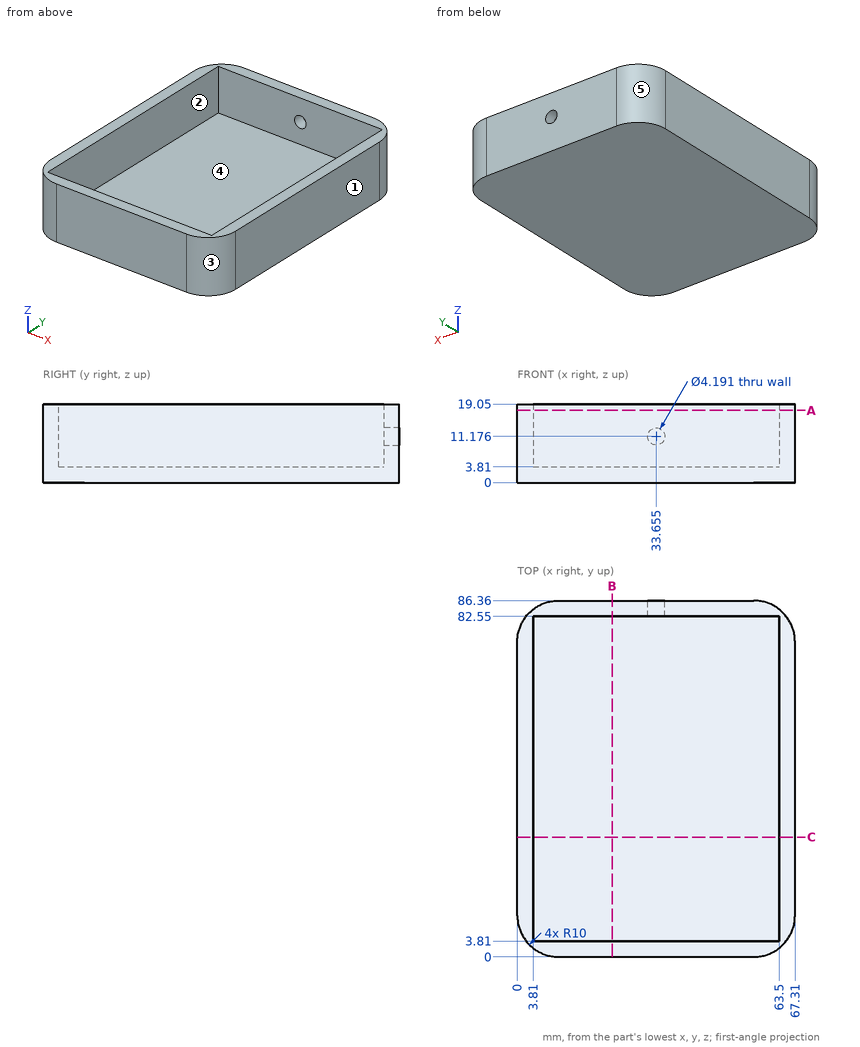
Can you work these out from the drawing? Everything is in mm from the part's minimum corner. A direction names the side the tool comes from. Round coordinates to 2 decimals unless told otherwise and drop trailing zeros. Write each loop counter-clockwise with the first axis right and the second up, starting at its lowest first coordinate (ties: lowest second). Pieces come first, ordered by that corner, then holes.
1. For the marked faces 1 and 2, which set-ups out of +Z, -Z, +X, -X, +Y, -Y let a thin tool reach every point of the face, with its end or its side?
2. Suppose I cut it at B-B (x = 23). List the corners of the cut face in (y, z) for me, and give its area (3 significant figures).
3. Suppose I cut it at A-A (z = 17.5). List the corners of the cut face in (x, y) for me, and give its area (3 significant figures).
4. If we mould it in two halves opening along X, with no side actions, what happens to the marked faces 3, 4 and 5? For each: released by +X, released by -X, zero draft, split by the parting line, or undercut.
5. I need wall thicknesses on L1, parallel to Y at x = 54, z = 18.25; L2, parallel to X at y = 74.5, z = 8; L3, parallel to Z at x = 58, y = 33. Which ranges of each line are inside material? Lowest first, please.
6. Suppose I cut it at C-C (y = 29). List the corners of the cut face in (x, z) for me, and give its area (3 significant figures).
Answer sheet:
1. face 1: +Z, -Z, +X, +Y, -Y
1. face 2: +Z
2. outline: (0, 0) - (86.36, 0) - (86.36, 19.05) - (82.55, 19.05) - (82.55, 3.81) - (3.81, 3.81) - (3.81, 19.05) - (0, 19.05) - close
2. area: 445 mm2
3. outline: (0, 10) arc R10 ccw to (10, 0) - (57.31, 0) arc R10 ccw to (67.31, 10) - (67.31, 76.36) arc R10 ccw to (57.31, 86.36) - (10, 86.36) arc R10 ccw to (0, 76.36) - close; hole (3.81, 3.81) - (63.5, 3.81) - (63.5, 82.55) - (3.81, 82.55) - close
3. area: 1,030 mm2
4. face 3: released by +X
4. face 4: undercut
4. face 5: released by -X
5. L1: y = 0 to 3.81, 82.55 to 86.36
5. L2: x = 0 to 3.81, 63.5 to 67.31
5. L3: z = 0 to 3.81
6. outline: (0, 0) - (67.31, 0) - (67.31, 19.05) - (63.5, 19.05) - (63.5, 3.81) - (3.81, 3.81) - (3.81, 19.05) - (0, 19.05) - close
6. area: 373 mm2
